from build123d import *

# Parameters (mm, degrees)
F0_W     = 13.208
F0_H     = 2.54
F0_W_2   = 5.842
F0_H_2   = 12.7
F1_DEPTH = 5.842


with BuildPart() as f1:
    # F0 (on Front) → F1 (new body)
    with BuildSketch(Plane.XZ):
        with Locations((-70.612, -24.13)):
            Rectangle(F0_W, F0_H)
        with Locations((-6.604, -24.13)):
            Rectangle(F0_W, F0_H)
        with Locations((-92.837, -12.7)):
            Rectangle(F0_W_2, F0_H_2)
        with Locations((15.621, -12.7)):
            Rectangle(F0_W_2, F0_H_2)
        Polygon((12.7, -6.35), (-89.916, -6.35), (-89.916, -19.05), (-89.916, -22.86), (-77.216, -22.86), (-64.008, -22.86), (-13.208, -22.86), (0, -22.86), (12.7, -22.86), (12.7, -19.05), align=None)
    extrude(amount=-F1_DEPTH)


solid = f1.part
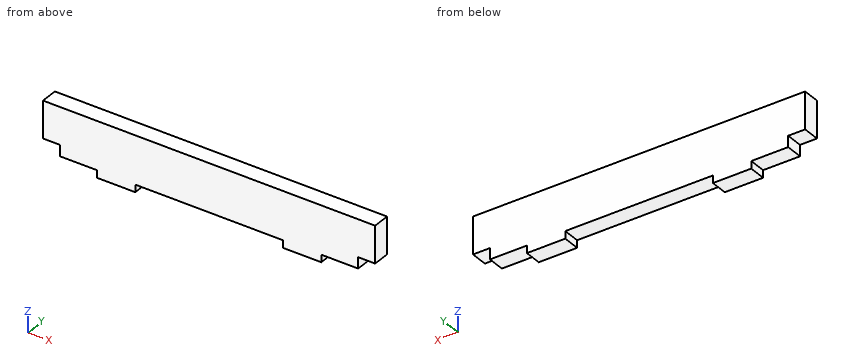
The model under review builds one solid part; all positions refer to its coordinate system, in mm. Coordinates: 2 decimals unless noted, no trailing zeros. Loops run counter-clockwise (first coordinate to the right, second up) from the corner with the lowest first, then second, coordinate; pieces in that order, holes last.
(1) Consider section C-C, the plane x = -43. Give the boundary of the cut face in (y, z).
Determined:
outline: (0, -22.86) - (5.84, -22.86) - (5.84, -6.35) - (0, -6.35) - close
(2) Consider section A-A, the plane y = 1.55. Give the boundary of the cut face in (x, z).
Determined:
outline: (-95.76, -19.05) - (-89.92, -19.05) - (-89.92, -22.86) - (-77.22, -22.86) - (-77.22, -25.4) - (-64.01, -25.4) - (-64.01, -22.86) - (-13.21, -22.86) - (-13.21, -25.4) - (0, -25.4) - (0, -22.86) - (12.7, -22.86) - (12.7, -19.05) - (18.54, -19.05) - (18.54, -6.35) - (-95.76, -6.35) - close
(3) Insertion check: P1, Ø1.8, axis at x = 15, y = 3, coming from the -Z side; P2, Ø1.3, axis at y = 3.5, z = -24, coming from the +X side; P3, Ø2, axis at y = 4, z = -24.5, coming from the -X side; P4, Ø5, axis at x = -77, z = -22.5, coming from the -Y side. Each pin has a flat end and moves straight along its axis. Give the tip position at first contact, or say it passes through.
Determined:
P1: stops at z = -19.05
P2: stops at x = 0
P3: stops at x = -77.22
P4: stops at y = 0
(4) Consider section B-B, the plane z = -20.5. Give the boundary of the cut face in (x, y), plus the area to 3 significant figures.
Determined:
outline: (-89.92, 0) - (12.7, 0) - (12.7, 5.84) - (-89.92, 5.84) - close
area: 599 mm2
(5) Wall thickness on L1, parallel to X at y = 4.1, z = -24; L2, parallel to X at y = 2.65, z = -21; L3, parallel to Z at x = -25.5, y = 0.35: over which ranges is each line inside the solid? List them lowest first.
Determined:
L1: x = -77.22 to -64.01, -13.21 to 0
L2: x = -89.92 to 12.7
L3: z = -22.86 to -6.35
